```python
from build123d import *

# Parameters (mm, degrees)
SKETCH1_W           = 60
SKETCH1_H           = 10
BOSS_EXTRUDE1_DEPTH = 17
CUT_EXTRUDE1_REACH  = 12
FILLET1_R           = 3
FILLET2_R           = 2
FILLET3_R           = 1


with BuildPart() as part:
    # Sketch1 → Boss-Extrude1 (new body)
    with BuildSketch(Plane.XY):
        with Locations((-89, -92.757283518)):
            Rectangle(SKETCH1_W, SKETCH1_H)
    extrude(amount=BOSS_EXTRUDE1_DEPTH)

    # Sketch2 → Cut-Extrude1 (cut, up to next)
    with BuildSketch(Plane.XZ.offset(97.757283518), mode=Mode.PRIVATE) as cut_extrude1_sk1:
        Polygon((-106.87061576, 17), (-112, 6), (-119, 6), (-119, 17), align=None)
    cut_extrude1_tool1 = extrude(cut_extrude1_sk1.sketch, amount=-CUT_EXTRUDE1_REACH, mode=Mode.PRIVATE) & part.part
    add(cut_extrude1_tool1.solids().sort_by_distance((-114.103037, -97.757284, 11.991593))[0], mode=Mode.SUBTRACT)
    # Sketch2 → Cut-Extrude1 (cut, up to next)
    with BuildSketch(Plane.XZ.offset(97.757283518), mode=Mode.PRIVATE) as cut_extrude1_sk2:
        Polygon((-59, 17), (-71.12938424, 17), (-66, 6), (-59, 6), align=None)
    cut_extrude1_tool2 = extrude(cut_extrude1_sk2.sketch, amount=-CUT_EXTRUDE1_REACH, mode=Mode.PRIVATE) & part.part
    add(cut_extrude1_tool2.solids().sort_by_distance((-63.896963, -97.757284, 11.991593))[0], mode=Mode.SUBTRACT)

    # Fillet1
    fillet1_edges = [part.edges().sort_by_distance(p)[0] for p in [
        (-66, -92.757283518, 6),
        (-71.12938424, -92.757283518, 17),
        (-106.87061576, -92.757283518, 17),
        (-112, -92.757283518, 6),
    ]]
    fillet(fillet1_edges, radius=FILLET1_R)

    # Fillet2
    fillet2_edges = [part.edges().sort_by_distance(p)[0] for p in [
        (-59, -97.757283518, 3),
        (-119, -97.757283518, 3),
        (-59, -87.757283518, 3),
        (-119, -87.757283518, 3),
    ]]
    fillet(fillet2_edges, radius=FILLET2_R)

    # Fillet3
    fillet3_edges = [part.edges().sort_by_distance(p)[0] for p in [
        (-62.544394609, -97.757283518, 6),
        (-65.700688043, -97.757283518, 6.469825663),
        (-68.56469212, -97.757283518, 11.5),
        (-71.428696197, -97.757283518, 16.530174337),
        (-115.455605391, -97.757283518, 6),
        (-89, -97.757283518, 17),
        (-112.299311957, -97.757283518, 6.469825663),
        (-106.571303803, -97.757283518, 16.530174337),
        (-109.43530788, -97.757283518, 11.5),
        (-59.585786438, -97.171497081, 6),
        (-59, -92.757283518, 6),
        (-62.544394609, -87.757283518, 6),
        (-59.585786438, -88.343069955, 6),
        (-65.700688043, -87.757283518, 6.469825663),
        (-68.56469212, -87.757283518, 11.5),
        (-118.414213562, -97.171497081, 6),
        (-71.428696197, -87.757283518, 16.530174337),
        (-119, -92.757283518, 6),
        (-115.455605391, -87.757283518, 6),
        (-118.414213562, -88.343069955, 6),
        (-89, -87.757283518, 17),
        (-112.299311957, -87.757283518, 6.469825663),
        (-106.571303803, -87.757283518, 16.530174337),
        (-109.43530788, -87.757283518, 11.5),
    ]]
    fillet(fillet3_edges, radius=FILLET3_R)


solid = part.part
```
Can you work these out from the model? Positions are in its coordinate system, mm. A direction names the side the tool comes from. Coordinates: 2 decimals unless noted, no trailing zeros. Loops run counter-clockwise (first coordinate to the right, second up) from the corner with the lowest first, then second, coordinate; pieces in that order, holes last.
Item 1: Which directions (+Z, -Z, +X, -X, +Y, -Y) give clear straight access to the entire face, cutting with the end or side of a thin tool? Please do faces 1 (the face through (-68.848, -88.058, 11.432)), 2 (the face through (-62.52, -97.46, 5.71)), 3 (the face through (-115.477, -88.058, 5.715)), 4 (the face through (-109.15, -97.46, 11.43)), 5 (the face through (-62, -93, 6)).
Answers below:
face 1: +Z, +X, +Y
face 2: +Z, +X, -Y
face 3: +Z, -X, +Y
face 4: +Z, -X, -Y
face 5: +Z, +X, +Y, -Y
Item 2: I'm going to push flat-ended pins straight in: pin 1 (1.5 mm diameter, centred on y = -89.5, z = 13, fed in from +X); pin 2 (2 mm diameter, centred on y = -91, z = 13.5, fed in from -X); pin 3 (1.2 mm diameter, centred on x = -117, y = -94.5, fed in from +Z). Where does each tip first touch, or does it pass through?
Answers below:
pin 1: stops at x = -68.91
pin 2: stops at x = -108.97
pin 3: stops at z = 6
Item 3: Please list where these lines run through material, in increasing order: L1, parallel to X at y = -88.25, z = 4.5; L2, parallel to X at y = -92, z = 6.5; L3, parallel to Z at x = -100.5, y = -88.5.
Answers below:
L1: x = -118.31 to -59.69
L2: x = -112.25 to -65.75
L3: z = 0 to 16.97
Item 4: Suppose I cut it at A-A (y = -93.25). Please give me the cut outline in (x, z).
Answers below:
outline: (-119, 0) - (-59, 0) - (-59, 5) arc R1 ccw to (-60, 6) - (-64.09, 6) arc R3 cw to (-66.81, 7.73) - (-70.32, 15.27) arc R3 ccw to (-73.04, 17) - (-104.96, 17) arc R3 ccw to (-107.68, 15.27) - (-111.19, 7.73) arc R3 cw to (-113.91, 6) - (-118, 6) arc R1 ccw to (-119, 5) - close
